Here's how the part is built. I have some questions about the finished solid (model axes, mm). A direction names the side the tool comes from. Give positions to 0.01 mm unless a question says otherwise; leave off trailing zeros. Order: outer loops, then holes, each group sorted by start corner. A loop starts at its lowest first (then second) coordinate and runs counter-clockwise, first axis right, second up. Notation, with made-up numbers: M 8,51 L 42,51 A11 cw 42,55 Z; hole C 51,17.25 d3. An arc over 180 degrees is marked long. Use CSV: the item, a comma, the result in double quotes. Start each with the question number.
```python
from build123d import *

# Parameters (mm, degrees)
EXTRUDE_1_DEPTH     = 45
SKETCH_2_R          = 3
CUT_EXTRUDE_1_DEPTH = 3
SKETCH_3_R          = 2.6
CUT_EXTRUDE_2_DEPTH = 3
SKETCH_4_R          = 1.6
CUT_EXTRUDE_3_DEPTH = 3


with BuildPart() as part:
    # ｽｹｯﾁ1 → ﾎﾞｽ - 押し出し1 (new body)
    with BuildSketch(Plane(origin=(0, 0, 0), x_dir=(0, 0, -1), z_dir=(1, 0, 0))):
        Polygon((-18, 40), (-18, 38), (0, 38), (0, 0), (2, 0), (2, 40), align=None)
    extrude(amount=EXTRUDE_1_DEPTH)

    # ｽｹｯﾁ2 → ｶｯﾄ - 押し出し1 (cut, through all)
    with BuildSketch(Plane.XZ.offset(-38)):
        with Locations((6, 6)):
            Circle(SKETCH_2_R)
        with Locations((39, 6)):
            Circle(SKETCH_2_R)
    extrude(amount=-CUT_EXTRUDE_1_DEPTH, mode=Mode.SUBTRACT)

    # ｽｹｯﾁ3 → ｶｯﾄ - 押し出し2 (cut, through all)
    with BuildSketch(Plane.XY):
        with Locations((22.5, 25)):
            Circle(SKETCH_3_R)
    extrude(amount=-CUT_EXTRUDE_2_DEPTH, mode=Mode.SUBTRACT)

    # ｽｹｯﾁ4 → ｶｯﾄ - 押し出し3 (cut, through all)
    with BuildSketch(Plane.XY):
        with Locations((13.5, 6)):
            Circle(SKETCH_4_R)
        with Locations((31.5, 6)):
            Circle(SKETCH_4_R)
    extrude(amount=-CUT_EXTRUDE_3_DEPTH, mode=Mode.SUBTRACT)


solid = part.part
```
Q1. We'd pull the mould along Y, two halves only. Please class faces 1 (the face through (23.9, 27.19, -0.99)), 2 (the face through (22, 40, 8)), 3 (the face through (45, 25, -1)): pulls with the +Y half, pulls with the -Y half, needs draft (parallel to the pull), parting line crosses it, or undercut.
Q2. Imagine slicing it at A-A, the plane x = 22.5. Please give me the cut outline in (y, z).
Q3. Imagine slicing it at D-D, the plane y = 25. Please give me the cut outline in (x, z), then the cut area to 3 significant figures.
Q4. I need wall thicknesses on line 1 (Y direction, x = 13.5, z = -1.15); line 2 (Y direction, x = 26, z = 10); line 3 (Z direction, x = 30, y = 3). Which ranges of each line are inside material? Lowest first, please. Write a range as [from, to].
Q5. Imagine slicing it at C-C, the plane z = 6. Please give me the cut outline in (x, y).
Q6. For P1, Ø9, axis at x = 28.5, z = 8.5, coming from the -Y side; P2, Ø2, axis at y = 28.5, z = 0.5, coming from the -X side; P3, Ø19, axis at x = 25, y = 11, coming from the +Z side, each with a flat end and sliding along its axis, tell me the tip position at first contact or that it passes through.
Q7. For faces 4 (the face through (22, 19, 0)), 5 (the face through (22, 20, -2)), which set-ups out of +Z, -Z, +X, -X, +Y, -Y let a thin tool reach every point of the face, with its end or its side?
Q8. Imagine slicing it at B-B, the plane y = 6. Please give me the cut outline in (x, z), then the cut area to 3 significant figures.
Reply:
1,face 1,"undercut"
1,face 2,"pulls with the +Y half"
1,face 3,"needs draft"
2,outline,"M 0,-2 L 22.4,-2 L 22.4,0 L 0,0 Z; M 27.6,-2 L 40,-2 L 40,18 L 38,18 L 38,0 L 27.6,0 Z"
3,outline,"M 0,-2 L 19.9,-2 L 19.9,0 L 0,0 Z; M 25.1,-2 L 45,-2 L 45,0 L 25.1,0 Z"
3,area,"79.6 mm^2"
4,line 1,"y = [0, 4.4], [7.6, 40]"
4,line 2,"y = [38, 40]"
4,line 3,"z = [-2, 0]"
5,outline,"M 0,38 L 3,38 L 3,40 L 0,40 Z; M 9,38 L 36,38 L 36,40 L 9,40 Z; M 42,38 L 45,38 L 45,40 L 42,40 Z"
6,P1,"stops at y = 38"
6,P2,"stops at x = 0"
6,P3,"stops at z = 0"
7,face 4,"+Z, +X, -X, -Y"
7,face 5,"-Z, +X, -X, +Y, -Y"
8,outline,"M 0,-2 L 11.9,-2 L 11.9,0 L 0,0 Z; M 15.1,-2 L 29.9,-2 L 29.9,0 L 15.1,0 Z; M 33.1,-2 L 45,-2 L 45,0 L 33.1,0 Z"
8,area,"77.2 mm^2"
